The listing builds one solid part. Answer for the finished solid, in the listing's coordinates (mm). A direction names the side the tool comes from. Coordinates: 2 decimals unless noted, no trailing zeros. Order: outer loops, then holes, each group sorted by start corner. A loop starts at its lowest first (then second) coordinate and runs counter-clockwise, first axis right, second up. Notation, with made-up numbers: (35.25, 12.5) -> (49.25, 12.5) arc R19 ccw to (49.25, 23.5) -> close; hole circle Ø1 at (30, -4). An arc over 180 degrees is marked (long way). Return JSON: item names as keys, results as strings.
Autodesk Inventor part; units mm, degrees
ref_plane "YZ Plane" through (0, 0, 0) normal (1, 0, 0) x (0, 1, 0)
ref_plane "XZ Plane" through (0, 0, 0) normal (0, 1, 0) x (-1, 0, 0)
ref_plane "XY Plane" through (0, 0, 0) normal (0, 0, 1) x (1, 0, 0)
sketch "Эскиз1" plane through (0, 0, 0) normal (0, 0, 1) x (1, 0, 0)
  circle A0 centre (0, 0) radius 80
  line L0 (26.5581, 0) -> (13.2791, -23)
  line L1 (13.2791, -23) -> (-13.2791, -23)
  line L2 (-13.2791, -23) -> (-26.5581, 0)
  line L3 (-26.5581, 0) -> (-13.2791, 23)
  line L4 (-13.2791, 23) -> (13.2791, 23)
  line L5 (13.2791, 23) -> (26.5581, 0)
  dimension "d49" = 160
  dimension "d50" = 46
extrude "Выдавливание1" add sketch "Эскиз1" along normal blind 4
sketch "Эскиз2" plane through (0, 0, 0) normal (0, 0, -1) x (-1, 0, 0)
  circle A0 centre (0, 0) radius 80
  line L0 (0, 80) -> (0, -80) construction
  line L1 (2, -80) -> (-2, -80)
  line L2 (-2, -80) -> (-2, 80)
  line L3 (-2, 80) -> (2, 80)
  line L4 (2, 80) -> (2, -80)
  line L5 (2, -80) -> (-2, 80) construction
  line L6 (-2, -80) -> (2, 80) construction
  line L7 (-2, 25) -> (2, 25)
  line L8 (-2, -25) -> (2, -25)
  point P0 (0, -25)
  point P1 (0, 80)
  point P2 (0, 25)
  dimension "d2" = 4
  dimension "d3" = 160
  dimension "d4" = 55
  dimension "d5" = 55
extrude "Выдавливание2" cut sketch "Эскиз2" against normal blind 10 contours L4 L7 L2 A0 | A0 L3 L4 | L4 L1 A0 | A0 L2 L8 L4 | A0 L2 L3 | L1 L2 A0
sketch "Эскиз4" plane through (0, 0, 4) normal (0, 0, 1) x (1, 0, 0)
  line L0 (56.2, 20) -> (38.2, 20)
  line L1 (37.2, 19) -> (37.2, -19)
  line L2 (57.2, -19) -> (57.2, 19)
  arc A0 (38.2, 20) -> (37.2, 19) centre (38.2, 19) ccw
  arc A1 (37.2, -19) -> (38.2, -20) centre (38.2, -19) ccw
  arc A2 (56.2, -20) -> (57.2, -19) centre (56.2, -19) ccw
  arc A3 (57.2, 19) -> (56.2, 20) centre (56.2, 19) ccw
  line L3 (44.9, -22) -> (49.5, -22)
  line L4 (49.7, -21.8) -> (49.7, -20.2)
  line L5 (49.7, -20) -> (47.2, -20) construction
  line L6 (44.7, -20.2) -> (44.7, -21.8)
  line L7 (49.7, -20) -> (44.7, -22) construction
  line L8 (47.2, -21) -> (47.2, -20) construction
  line L9 (0, 0) -> (112.2307, 0) construction
  line L10 (56.9071, 19.7071) -> (37.4929, -19.7071) construction
  line L11 (37.4929, 19.7071) -> (56.9071, -19.7071) construction
  line L12 (47.2, 20) -> (47.2, -20) construction
  line L13 (38.2, -20) -> (44.5, -20)
  line L14 (49.9, -20) -> (56.2, -20)
  arc A4 (49.9, -20) -> (49.7, -20.2) centre (49.9, -20.2) ccw
  arc A5 (44.7, -20.2) -> (44.5, -20) centre (44.5, -20.2) ccw
  arc A6 (44.7, -21.8) -> (44.9, -22) centre (44.9, -21.8) ccw
  arc A7 (49.5, -22) -> (49.7, -21.8) centre (49.5, -21.8) ccw
  line L15 (0, 0) -> (0, 111.2909) construction
  line L16 (47.2, -20) -> (47.2, -24.7856) construction
  point P0 (47.3361, 0)
  point P1 (49.7, -22)
  point P2 (44.7, -20)
  point P3 (47.2, 0)
  dimension "d35" = 1
  dimension "d40" = 5
  dimension "d41" = 2
  dimension "d42" = 20
  dimension "d44" = 37.2
  dimension "d45" = 0.2
  dimension "d46" = 38
extrude "Выдавливание4" cut sketch "Эскиз4" against normal blind 10
sketch "Эскиз6" plane through (0, 0, 4) normal (0, 0, 1) x (1, 0, 0)
  circle A0 centre (42.2, -25) radius 1.5
  circle A1 centre (52.2, -25) radius 1.5
  line L0 (42.2, -25) -> (52.2, -25) construction
  line L1 (52.2, -25) -> (52.2, 25) construction
  line L2 (52.2, 25) -> (42.2, 25) construction
  line L3 (42.2, 25) -> (42.2, -25) construction
  line L4 (42.2, -25) -> (52.2, 25) construction
  circle A2 centre (42.2, 25) radius 1.5
  circle A3 centre (52.2, 25) radius 1.5
  arc A4 (38.2, 20) -> (37.2, 19) centre (38.2, 19) ccw
  arc A5 (56.2, -20) -> (57.2, -19) centre (56.2, -19) ccw
  line L5 (38.2, 19) -> (56.2, -19) construction
  point P0 (0, 0)
  point P1 (47.2, 0)
  dimension "d15" = 3
  dimension "d16" = 50
  dimension "d17" = 10
  dimension "d20" = 3
  dimension "d21" = 3
  dimension "d22" = 3
extrude "Выдавливание5" cut sketch "Эскиз6" against normal blind 10
sketch "Эскиз8" plane through (0, 0, 4) normal (0, 0, 1) x (1, 0, 0)
  circle A0 centre (-32, 44.908) radius 2.55 construction
  circle A1 centre (-12, 44.908) radius 2.55 construction
  circle A2 centre (12, 44.908) radius 2.55 construction
  circle A3 centre (32, 44.908) radius 2.55 construction
  circle A4 centre (32, -44.908) radius 2.55 construction
  circle A5 centre (12, -44.908) radius 2.55 construction
  circle A6 centre (-32, -44.908) radius 2.55 construction
  circle A7 centre (-12, -44.908) radius 2.55 construction
  circle A8 centre (-32, 44.908) radius 1.95
  circle A9 centre (-12, 44.908) radius 1.95
  circle A10 centre (12, 44.908) radius 1.95
  circle A11 centre (32, 44.908) radius 1.95
  circle A12 centre (-32, -44.908) radius 1.95
  circle A13 centre (-12, -44.908) radius 1.95
  circle A14 centre (12, -44.908) radius 1.95
  circle A15 centre (32, -44.908) radius 1.95
  point P0 (0, 0)
  dimension "d23" = 3.9
  dimension "d24" = 3.9
  dimension "d25" = 3.9
  dimension "d26" = 3.9
  dimension "d27" = 3.9
  dimension "d28" = 3.9
  dimension "d29" = 3.9
  dimension "d30" = 3.9
extrude "Выдавливание6" cut sketch "Эскиз8" against normal blind 10
sketch "Эскиз9" plane through (0, 0, 0) normal (0, 0, -1) x (-1, 0, 0)
  circle A0 centre (-23.3827, -13.5) radius 2
  circle A1 centre (-23.3827, 13.5) radius 2
  circle A2 centre (23.3827, 13.5) radius 2
  circle A3 centre (23.3827, -13.5) radius 2
extrude "Выдавливание7" cut sketch "Эскиз9" against normal blind 10
properties part number "лицо1"
1. Consider line 1 (Y direction, x = -12, z = 0.95); line 2 (X direction, y = -46, z = 2.05); line 3 (X direction, y = -9, z = 0.5). Determine where each line is inside the solid, lowest interval first. Write a range as from..to.
Answer block:
{"line 1": "y = -79.09..-46.86, -42.96..-23, 23..42.96, 46.86..79.09", "line 2": "x = -65.45..-33.62, -30.38..-13.62, -10.38..-2, 2..10.38, 13.62..30.38, 33.62..65.45", "line 3": "x = -79.49..-21.36, 21.36..37.2, 57.2..79.49"}
2. Each of these flat-tipped pins is pushed along its axis until it touches: pin 1 Ø1.5 at (x, z) = (35.5, 0.5) entering from -Y; pin 2 Ø1.8 at (x, y) = (52.2, -25) entering from +Z; pin 3 Ø1.2 at (x, z) = (0.5, 2.5) entering from +Y; pin 4 Ø0.5 at (y, z) = (-21.5, 2) entering from +X. Where does it stop, or does it pass through?
Answer block:
{"pin 1": "stops at y = -72.06", "pin 2": "passes through", "pin 3": "stops at y = 25", "pin 4": "stops at x = 77.13"}
3. The part is cut by section A-A on x = 0. Give the vertices of the cut face in (y, z).
Answer block:
{"outline": "(-25, 0) -> (-23, 0) -> (-23, 4) -> (-25, 4) -> close; (23, 0) -> (25, 0) -> (25, 4) -> (23, 4) -> close"}
4. The part is cut by section B-B on y = -57. Give the vertices of the cut face in (x, z).
Answer block:
{"outline": "(-56.13, 0) -> (-2, 0) -> (-2, 4) -> (-56.13, 4) -> close; (2, 0) -> (56.13, 0) -> (56.13, 4) -> (2, 4) -> close"}
5. The part is cut by section D-D on z = 0.6. Give the number of separate pieces and of enclosed holes in the cut face, and give its area (3 significant figures).
Answer block:
{"separate pieces": "1", "enclosed holes": "18", "area": "16,900 mm2"}
6. The part is cut by section C-C on y = 6. Give the vertices of the cut face in (x, z).
Answer block:
{"outline": "(-79.77, 0) -> (-23.09, 0) -> (-23.09, 4) -> (-79.77, 4) -> close; (23.09, 0) -> (37.2, 0) -> (37.2, 4) -> (23.09, 4) -> close; (57.2, 0) -> (79.77, 0) -> (79.77, 4) -> (57.2, 4) -> close"}
7. For faces 1 (the face through (-19, -17, 0)), 2 (the face through (-2, 53, 2)), 3 (the face through (19.826, 11.661, 1.972)), determine the directions among +Z, -Z, +X, -X, +Y, -Y from which every point of the face is accessible in a straight line to the end or side of a thin tool.
Answer block:
{"face 1": "-Z, +X, -X, +Y, -Y", "face 2": "+Z, -Z, +Y", "face 3": "+Z, -Z"}
8. Determine the mould class of faces 4 (the face through (-79.98, -1.73, 1.97)), 5 (the face through (0, -25, 2)), 6 (the face through (11.6, 43, 2)) for opening direction Y: pulls with the +Y half, pulls with the -Y half, needs draft (parallel to the pull), parting line crosses it, or undercut.
Answer block:
{"face 4": "parting line crosses it", "face 5": "pulls with the -Y half", "face 6": "undercut"}
